from build123d import *

# Parameters (mm, degrees)
SKETCH1_W           = 100
SKETCH1_H           = 100
BOSS_EXTRUDE1_DEPTH = 5
SKETCH2_4_R         = 8.75
SKETCH3_3_R         = 6.25
SKETCH2_5_R         = 8.75
SKETCH3_4_R         = 6.25
SKETCH2_6_R         = 8.75
SKETCH3_5_R         = 6.25


with BuildPart() as part:
    # Sketch1 → Boss-Extrude1 (new, symmetric)
    with BuildSketch(Plane(origin=(0, 0, 0), x_dir=(1, 0, 0), z_dir=(0, 1, 0))):
        Rectangle(SKETCH1_W, SKETCH1_H)
    extrude(amount=BOSS_EXTRUDE1_DEPTH, both=True)

    # Loft1: read off the stored shape, not the designer's step
    # Loft1: loft between two sections, ruled curve by curve
    loft1_from = [
        Edge.make_bspline([(-44.368650168, -5, -32.418615185), (-59.531419798, -5, -41.15591552), (-50.794119462, -5, -56.31868515), (-35.631349832, -5, -47.581384815), (-20.468580202, -5, -38.84408448), (-29.205880538, -5, -23.68131485), (-44.368650168, -5, -32.418615185)], [0, 0, 0, 0, 0.5, 0.5, 0.5, 1, 1, 1, 1], 3, [1, 0.333333333, 0.333333333, 1, 0.333333333, 0.333333333, 1]),
    ]
    loft1_to = [
        Edge.make_bspline([(-41.905194087, -75, -34.047459745), (-53.810274598, -75, -37.857847919), (-49.999886423, -75, -49.76292843), (-38.094805913, -75, -45.952540255), (-26.189725402, -75, -42.142152081), (-30.000113577, -75, -30.23707157), (-41.905194087, -75, -34.047459745)], [0, 0, 0, 0, 0.5, 0.5, 0.5, 1, 1, 1, 1], 3, [1, 0.333333333, 0.333333333, 1, 0.333333333, 0.333333333, 1]),
    ]
    loft1 = Solid(Shell([*[Face.make_surface_from_curves(loft1_from[k], loft1_to[k]) for k in range(1)], Face(Wire(loft1_from)), Face(Wire(loft1_to))]))
    add(loft1)

    # Sketch2<4> → Loft2 section 0
    with BuildSketch(Plane.XZ.offset(5)):
        with Locations((-40, 40)):
            Circle(SKETCH2_4_R)
    # Sketch3<3> → Loft2 section 1
    with BuildSketch(Plane(origin=(0, -75, 0), x_dir=(1, 0, 0), z_dir=(0, 1, 0))):
        with Locations((-40, -40)):
            Circle(SKETCH3_3_R)
    loft()

    # Sketch2<5> → Loft3 section 0
    with BuildSketch(Plane.XZ.offset(5)):
        with Locations((40, 40)):
            Circle(SKETCH2_5_R)
    # Sketch3<4> → Loft3 section 1
    with BuildSketch(Plane(origin=(0, -75, 0), x_dir=(1, 0, 0), z_dir=(0, 1, 0))):
        with Locations((40, -40)):
            Circle(SKETCH3_4_R)
    loft()

    # Sketch2<6> → Loft4 section 0
    with BuildSketch(Plane.XZ.offset(5)):
        with Locations((40, -40)):
            Circle(SKETCH2_6_R)
    # Sketch3<5> → Loft4 section 1
    with BuildSketch(Plane(origin=(0, -75, 0), x_dir=(1, 0, 0), z_dir=(0, 1, 0))):
        with Locations((40, 40)):
            Circle(SKETCH3_5_R)
    loft()


solid = part.part
Model file for the job. Use its own axes, mm. A direction names the side the tool comes from. Round coordinates to 2 decimals unless told otherwise and drop trailing zeros. Order: outer loops, then holes, each group sorted by start corner. A loop starts at its lowest first (then second) coordinate and runs counter-clockwise, first axis right, second up.
(1) Drill centre lines: line 1 (Y direction, x = -24, z = -10); line 2 (Z direction, x = 32.5, y = -14.5); line 3 (X direction, y = -60, z = -37). Where is each one in solid material? Low to high.
(2) 3-axis set-ups, long thin cutter, end or side, ignore diameter. For faces 4 (the face through (7, -5, -4)), 5 (the face through (-1, 5, -1)): which of +Z, -Z, +X, -X, +Y, -Y reach the whole face in a straight line?
(3) Pin check, flat tips, straight feed: pin 1 (5 mm diameter, centred on y = -28, z = -30.5, fed in from +X); pin 2 (8 mm diameter, centred on x = -17.5, z = -36.5, fed in from -Y); pin 3 (2 mm diameter, centred on y = -51.5, z = 30.5, fed in from +X). Stop position of each tip, or through.
(4) Pull direction Z, two halves, no side cores. Call faces 1 (the face through (46.91, -40.49, -42.87)), 2 (the face through (-1, 0, 50)), 3 (the face through (-40, -75, 40)): released by +Z, released by -Z, zero draft, split by the parting line, or undercut.
(5) Band-saw the part on B-B (z = 3). List the corners of the cut face in (x, y).
(6) Band-saw the part on A-A (x = 40). List the corners of the cut face in (y, z), then the cut area to 3 significant figures.
(7) Band-saw the part on C-C (x = 0). List the corners of the cut face in (y, z), then the cut area to 3 significant figures.
Verdict:
1. line 1: y = -5 to 5
1. line 2: z = -43.81 to -36.19, 36.19 to 43.81
1. line 3: x = -46.05 to -33.95, 33.91 to 46.09
2. face 4: -Y
2. face 5: +Z, -Z, +X, -X, +Y
3. pin 1: stops at x = 43.73
3. pin 2: stops at y = -5
3. pin 3: passes through
4. face 1: undercut
4. face 2: released by +Z
4. face 3: zero draft
5. outline: (-50, -5) - (50, -5) - (50, 5) - (-50, 5) - close
6. outline: (-75, -46.25) - (-5, -48.75) - (-5, -50) - (5, -50) - (5, 50) - (-5, 50) - (-5, 48.75) - (-75, 46.25) - (-75, 33.75) - (-5, 31.25) - (-5, -31.25) - (-75, -33.75) - close
6. area: 3,100 mm2
7. outline: (-5, -50) - (5, -50) - (5, 50) - (-5, 50) - close
7. area: 1,000 mm2
